Autodesk Fusion 360 part; units mm, degrees
sketch "スケッチ1" plane through (0, 0, 0) normal (0, 0, 1) x (1, 0, 0)
  line L0 (240.4841, -190.269) -> (351.6841, -190.269)
  line L1 (240.4841, -187.969) -> (351.6841, -187.969)
  line L2 (351.6841, -115.269) -> (240.4841, -115.269)
  line L3 (351.6841, -117.569) -> (240.4841, -117.569)
  arc A0 (233.5841, -183.369) -> (240.4841, -190.269) centre (240.4841, -183.369) ccw
  arc A1 (235.8841, -183.369) -> (240.4841, -187.969) centre (240.4841, -183.369) ccw
  arc A2 (240.4841, -115.269) -> (233.5841, -122.169) centre (240.4841, -122.169) ccw
  line L4 (233.5841, -122.169) -> (233.5841, -183.369)
  line L5 (235.8841, -122.169) -> (235.8841, -183.369)
  arc A3 (240.4841, -117.569) -> (235.8841, -122.169) centre (240.4841, -122.169) ccw
  arc A4 (351.6841, -190.269) -> (358.5841, -183.369) centre (351.6841, -183.369) ccw
  arc A5 (351.6841, -187.969) -> (356.2841, -183.369) centre (351.6841, -183.369) ccw
  line L6 (358.5841, -183.369) -> (358.5841, -122.169)
  line L7 (356.2841, -183.369) -> (356.2841, -122.169)
  arc A6 (358.5841, -122.169) -> (351.6841, -115.269) centre (351.6841, -122.169) ccw
  arc A7 (356.2841, -122.169) -> (351.6841, -117.569) centre (351.6841, -122.169) ccw
  point P0 (296.0841, -152.769)
extrude "押し出し1" add sketch "スケッチ1" along normal blind 100
Read the model definition and answer for the solid it produces. Units are mm, in the model's axes. A direction names the side the tool comes from. Coordinates: 2 decimals unless noted, no trailing zeros. Order: outer loops, then holes, each group sorted by start corner. A loop starts at its lowest first (then second) coordinate and runs counter-clockwise, first axis right, second up. Notation, with made-up numbers: M 25,-32 L 53,-32 A23 cw 53,1 Z; hole C -34,54.25 d2. An arc over 180 degrees is marked long. Put each result on its own line as item: value. Start each with the question number.
Item 1: For faces 4 (the face through (354.97, -186.59, 49.3)), 5 (the face through (277, -189, 0)), determine the directions among +Z, -Z, +X, -X, +Y, -Y from which every point of the face is accessible in a straight line to the end or side of a thin tool.
Item 2: Section A-A, the plane y = -151 is taken. Determine the outline of the cut face in (x, z).
Item 3: Consider probe 1 along Y at (x, z) = (308.5, 21); probe 2 along X at (y, z) = (-132, 9); probe 3 along X at (y, z) = (-186, 76). Determine where each line is inside the solid, lowest interval first. Write a range as [from, to].
Item 4: Section B-B, the plane x = 277.5 is taken. Determine the outline of the cut face in (y, z), plus the area to 3 significant figures.
Item 5: The mould has two halves that part along X. Classify faces 1 (the face through (233.584, -152, 49)), 2 (the face through (295, -190.269, 49)), 3 (the face through (297, -117.569, 49)): +X half, -X half, draft (parallel to the pull), parting line (faces both ways), or undercut.
Item 6: Section C-C, the plane z = 37.5 is taken. Determine the outline of the cut face in (x, y).
Computed:
1. face 4: +Z, -Z
1. face 5: -Z, +X, -X, +Y, -Y
2. outline: M 233.58,0 L 235.88,0 L 235.88,100 L 233.58,100 Z; M 356.28,0 L 358.58,0 L 358.58,100 L 356.28,100 Z
3. probe 1: y = [-190.27, -187.97], [-117.57, -115.27]
3. probe 2: x = [233.58, 235.88], [356.28, 358.58]
3. probe 3: x = [234.11, 236.71], [355.46, 358.06]
4. outline: M -190.27,0 L -187.97,0 L -187.97,100 L -190.27,100 Z; M -117.57,0 L -115.27,0 L -115.27,100 L -117.57,100 Z
4. area: 460 mm2
5. face 1: -X half
5. face 2: draft
5. face 3: undercut
6. outline: M 233.58,-183.37 A6.9 ccw 240.48,-190.27 L 351.68,-190.27 A6.9 ccw 358.58,-183.37 L 358.58,-122.17 A6.9 ccw 351.68,-115.27 L 240.48,-115.27 A6.9 ccw 233.58,-122.17 Z; hole M 235.88,-183.37 A4.6 ccw 240.48,-187.97 L 351.68,-187.97 A4.6 ccw 356.28,-183.37 L 356.28,-122.17 A4.6 ccw 351.68,-117.57 L 240.48,-117.57 A4.6 ccw 235.88,-122.17 Z
